```python
from build123d import *

# Parameters (mm, degrees)
SKETCH_2_R          = 1
CUT_EXTRUDE_1_DEPTH = 8


with BuildPart() as part:
    # 草图1 → 旋转2 (revolve)
    with BuildSketch(Plane(origin=(0, 0, 0), x_dir=(1, 0, 0), z_dir=(0, 1, 0)), mode=Mode.PRIVATE) as revolve_2_sk:
        Polygon((11.5, 0), (11.5, 2.75), (0, 2.75), (0, 5), (-8, 5), (-26.5, 3.25), (-26.5, 0), align=None)
    revolve(revolve_2_sk.sketch.rotate(Axis((-52.597365488, 0, 0), (1, 0, 0)), 180), axis=Axis((-52.597365488, 0, 0), (1, 0, 0)))

    # 草图2 → 切除-拉伸1 (cut)
    with BuildSketch(Plane(origin=(11.5, 0, 0), x_dir=(0, 0, -1), z_dir=(1, 0, 0))):
        Circle(SKETCH_2_R)
    extrude(amount=-CUT_EXTRUDE_1_DEPTH, mode=Mode.SUBTRACT)


solid = part.part
```
CAD build for the part. Positions are in the model's coordinates, mm. A direction names the side the tool comes from. Give positions to 0.01 mm unless a question says otherwise; leave off trailing zeros. Write each loop counter-clockwise with the first axis right and the second up, starting at its lowest first coordinate (ties: lowest second). Pieces come first, ordered by that corner, then holes. Notation, with made-up numbers: M -13.75,-8.5 L 8.25,-8.5 A17 cw 8.25,2.5 Z; hole C 39,83.5 d4. An arc over 180 degrees is marked long. Return JSON: item names as keys, results as strings. Group by question number.
(1) Flat gauge pins, fed straight in: pin 1 Ø4 at (x, z) = (-22.5, 3) entering from +Y; pin 2 Ø1.5 at (x, y) = (-22.5, 0.5) entering from +Z; pin 3 Ø3 at (x, z) = (-17.5, -1) entering from -Y. Where does each tip first touch, or does it go through?
(2) Band-saw the part on A-A (y = 0). Give the cut face in (x, z), and give its area (3 significant figures).
(3) Band-saw the part on C-C (x = -6). Give the cut face in (y, z), and give its area (3 significant figures).
(4) 3-axis set-ups, long thin cutter, end or side, ignore diameter. For faces 5 (the face through (5.67, 2.685, -0.596)), 6 (the face through (-17.38, -1.24, 3.92)): which of +Z, -Z, +X, -X, +Y, -Y reach the whole face in a straight line?
(5) Drill centre lines: L1, parallel to Y at x = 5.5, z = 0; L2, parallel to X at y = -1, z = -2.75; L3, parallel to Y at x = 8.5, z = -2.5. Where is each one in solid material? Low to high. Write a range as [from, to].
(6) Mould opens along Z. For faces 1 (the face through (3.5, 0, 0)), 2 (the face through (8, -1, 0)), 3 (the face through (-4, 0, -5)), 4 (the face through (-26.5, 0, 0)) say: pulls with the +Z half, pulls with the -Z half, needs draft (parallel to the pull), parting line crosses it, or undercut.
(7) Band-saw the part on D-D (x = -11.5). Give the cut face in (y, z).
Entries:
{
 "1": {"pin 1": "stops at y = 3.52", "pin 2": "stops at z = 3.69", "pin 3": "stops at y = -4.22"},
 "2": {"outline": "M -26.5,-3.25 L -8,-5 L 0,-5 L 0,-2.75 L 11.5,-2.75 L 11.5,-1 L 3.5,-1 L 3.5,1 L 11.5,1 L 11.5,2.75 L 0,2.75 L 0,5 L -8,5 L -26.5,3.25 Z", "area": "280 mm^2"},
 "3": {"outline": "C 0,0 d10", "area": "78.5 mm^2"},
 "4": {"face 5": "+X", "face 6": "-X"},
 "5": {"L1": "y = [-2.75, -1], [1, 2.75]", "L2": "x = [-26.5, 0]", "L3": "y = [-1.15, 1.15]"},
 "6": {"face 1": "undercut", "face 2": "undercut", "face 3": "parting line crosses it", "face 4": "needs draft"},
 "7": {"outline": "C 0,0 d9.34"}
}
